Source: CAD feature listing. Evaluate the final solid. Frame: model axes, mm. Give positions to 0.01 mm unless a question says otherwise; leave off trailing zeros. Write each loop counter-clockwise with the first axis right and the second up, starting at its lowest first coordinate (ties: lowest second). Pieces come first, ordered by that corner, then holes. Notation, with made-up numbers: (-26, -37.5) -> (1, -37.5) arc R22 cw to (1, -5.5) -> close; hole circle Ø6 at (45, 6.25). An arc over 180 degrees is marked (long way). Write item = value, one per line.
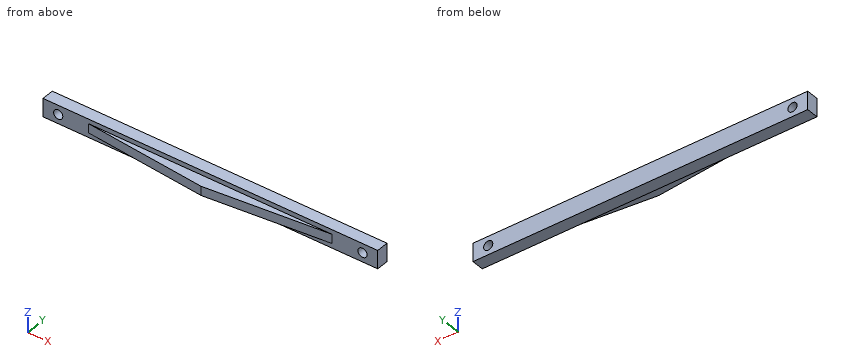
from build123d import *

# Parameters (mm, degrees)
SKETCH1_W                = 110
SKETCH1_H                = 4
BOSS_EXTRUDE1_DEPTH      = 3
BOSS_EXTRUDE2_DEPTH      = 1.5
F_3_0_3_DIAMETER_HOLE1_D = 3


with BuildPart() as part:
    # Sketch1 → Boss-Extrude1 (new, symmetric)
    with BuildSketch(Plane.XY):
        Rectangle(SKETCH1_W, SKETCH1_H)
    extrude(amount=BOSS_EXTRUDE1_DEPTH, both=True)

    # Sketch2 → Boss-Extrude2 (add, symmetric)
    with BuildSketch(Plane.XY):
        Polygon((-40, -2), (0, -6), (40, -2), align=None)
    extrude(amount=BOSS_EXTRUDE2_DEPTH, both=True)

    # Ø3.0 (3) Diameter Hole1 (through all)
    with Locations(Plane(origin=(0, 2, 0), x_dir=(1, 0, 0), z_dir=(0, 1, 0))):
        with Locations((-50, 0), (50, 0)):
            Hole(F_3_0_3_DIAMETER_HOLE1_D / 2)


solid = part.part
(1) Material intervals for line 1 (Z direction, x = 50, y = 0.3); line 2 (Z direction, x = 27, y = -3); line 3 (X direction, y = -1.25, z = -0.95), sorted ascending.
Values follow:
line_1 = -3 to -1.5, 1.5 to 3
line_2 = -1.5 to 1.5
line_3 = -55 to -51.16, -48.84 to 48.84, 51.16 to 55
(2) Section query A-A (x = -50). Return loops of the section in (y, z).
Values follow:
outline = (-2, -3) -> (2, -3) -> (2, -1.5) -> (-2, -1.5) -> close; (-2, 1.5) -> (2, 1.5) -> (2, 3) -> (-2, 3) -> close
(3) Section query B-B (z = 0). Return loops of the section in (x, y), plus the area to 3 significant figures.
Values follow:
outline = (-55, -2) -> (-51.5, -2) -> (-51.5, 2) -> (-55, 2) -> close; (-48.5, -2) -> (-40, -2) -> (0, -6) -> (40, -2) -> (48.5, -2) -> (48.5, 2) -> (-48.5, 2) -> close; (51.5, -2) -> (55, -2) -> (55, 2) -> (51.5, 2) -> close
area = 576 mm2
(4) First-contact query: pin 1 (1.2 mm diameter, centred on x = -14, y = -4, fed in from -Z); pin 2 (4.5 mm diameter, centred on x = 0.5, y = -4.5, fed in from +Z). Flat tips, straight axial feed; report the tip coordinate or a pass-through.
Values follow:
pin_1 = -1.5
pin_2 = 1.5
(5) Section query C-C (x = -36). Return loops of the section in (y, z), plus the area to 3 significant figures.
Values follow:
outline = (-2.4, -1.5) -> (-2, -1.5) -> (-2, -3) -> (2, -3) -> (2, 3) -> (-2, 3) -> (-2, 1.5) -> (-2.4, 1.5) -> close
area = 25.2 mm2
(6) Section query D-D (y = -0.75). Return loops of the section in (x, z).
Values follow:
outline = (-55, -3) -> (55, -3) -> (55, 3) -> (-55, 3) -> close; hole circle Ø3 at (-50, 0); hole circle Ø3 at (50, 0)
